Autodesk Inventor part; units mm, degrees
ref_plane "mss_or_XY" through (0, 0, 0) normal (1, 0, 0) x (0, 0, -1)
ref_plane "mss_or_YZ" through (0, 0, 0) normal (0, 0, -1) x (0, 1, 0)
ref_plane "mss_or_ZX" through (0, 0, 0) normal (0, 1, 0) x (1, 0, 0)
sketch "Sketch_3" plane through (0, 0, 0) normal (0, 0, 1) x (1, 0, 0)
  line L0 (6, 0) -> (0, 0)
  line L1 (0, 7.964) -> (0.135, 7.964)
  line L2 (0.135, 7.964) -> (0.135, 7.58)
  line L3 (0.135, 7.58) -> (1.5901, 7.58)
  arc A0 (4.4099, 7.58) -> (1.5901, 7.58) centre (3, 6.5) ccw
  line L4 (4.4099, 7.58) -> (5.865, 7.58)
  line L5 (5.865, 7.58) -> (5.865, 7.964)
  line L6 (5.865, 7.964) -> (6, 7.964)
  line L7 (6, 7.964) -> (6, 9.2)
  arc A1 (6, 9.2) -> (5.7, 9.5) centre (5.7, 9.2) ccw
  line L8 (5.7, 9.5) -> (0.3, 9.5)
  arc A2 (0.3, 9.5) -> (0, 9.2) centre (0.3, 9.2) ccw
  line L9 (0, 9.2) -> (0, 7.964)
revolve "Revolution1" add sketch "Sketch_3" angle 360 about axis through (6, 0, 0) along (1, 0, 0)
ref_plane "mss_or_XY" through (0, 0, 0) normal (1, 0, 0) x (0, 0, -1)
ref_plane "mss_or_YZ" through (0, 0, 0) normal (0, 0, -1) x (0, 1, 0)
ref_plane "mss_or_ZX" through (0, 0, 0) normal (0, 1, 0) x (1, 0, 0)
ref_plane "mss_or11_XY" through (6, 0, 0) normal (1, 0, 0) x (0, 0, -1)
ref_plane "mss_or11_YZ" through (6, 0, 0) normal (0, 0, -1) x (0, 1, 0)
ref_plane "mss_or11_ZX" through (6, 0, 0) normal (0, 1, 0) x (1, 0, 0)
ref_plane "mss_or2_1_XY" through (3, 6.5, 0) normal (1, 0, 0) x (0, 0, -1)
ref_plane "mss_or2_1_YZ" through (3, 6.5, 0) normal (0, 0, -1) x (0, 1, 0)
ref_plane "mss_or2_1_ZX" through (3, 6.5, 0) normal (0, 1, 0) x (1, 0, 0)
ref_plane "mss_or2_2_XY" through (3, 4.0527, 5.0819) normal (1, 0, 0) x (0, 0, -1)
ref_plane "mss_or2_2_YZ" through (3, 4.0527, 5.0819) normal (0, 0, -1) x (0, 1, 0)
ref_plane "mss_or2_2_ZX" through (3, 4.0527, 5.0819) normal (0, 1, 0) x (1, 0, 0)
ref_plane "mss_or2_3_XY" through (3, -1.4464, 6.337) normal (1, 0, 0) x (0, 0, -1)
ref_plane "mss_or2_3_YZ" through (3, -1.4464, 6.337) normal (0, 0, -1) x (0, 1, 0)
ref_plane "mss_or2_3_ZX" through (3, -1.4464, 6.337) normal (0, 1, 0) x (1, 0, 0)
ref_plane "mss_or2_4_XY" through (3, -5.8563, 2.8202) normal (1, 0, 0) x (0, 0, -1)
ref_plane "mss_or2_4_YZ" through (3, -5.8563, 2.8202) normal (0, 0, -1) x (0, 1, 0)
ref_plane "mss_or2_4_ZX" through (3, -5.8563, 2.8202) normal (0, 1, 0) x (1, 0, 0)
ref_plane "mss_or2_5_XY" through (3, -5.8563, -2.8202) normal (1, 0, 0) x (0, 0, -1)
ref_plane "mss_or2_5_YZ" through (3, -5.8563, -2.8202) normal (0, 0, -1) x (0, 1, 0)
ref_plane "mss_or2_5_ZX" through (3, -5.8563, -2.8202) normal (0, 1, 0) x (1, 0, 0)
ref_plane "mss_or2_6_XY" through (3, -1.4464, -6.337) normal (1, 0, 0) x (0, 0, -1)
ref_plane "mss_or2_6_YZ" through (3, -1.4464, -6.337) normal (0, 0, -1) x (0, 1, 0)
ref_plane "mss_or2_6_ZX" through (3, -1.4464, -6.337) normal (0, 1, 0) x (1, 0, 0)
ref_plane "mss_or2_7_XY" through (3, 4.0527, -5.0819) normal (1, 0, 0) x (0, 0, -1)
ref_plane "mss_or2_7_YZ" through (3, 4.0527, -5.0819) normal (0, 0, -1) x (0, 1, 0)
ref_plane "mss_or2_7_ZX" through (3, 4.0527, -5.0819) normal (0, 1, 0) x (1, 0, 0)
ref_plane "mss_or21_1_XY" through (3, 6.5, 0) normal (1, 0, 0) x (0, 0, -1)
ref_plane "mss_or21_1_YZ" through (3, 6.5, 0) normal (0, 0, -1) x (0, 1, 0)
ref_plane "mss_or21_1_ZX" through (3, 6.5, 0) normal (0, 1, 0) x (1, 0, 0)
ref_plane "mss_or21_2_XY" through (3, 4.0527, 5.0819) normal (1, 0, 0) x (0, 0, -1)
ref_plane "mss_or21_2_YZ" through (3, 4.0527, 5.0819) normal (0, 0, -1) x (0, 1, 0)
ref_plane "mss_or21_2_ZX" through (3, 4.0527, 5.0819) normal (0, 1, 0) x (1, 0, 0)
ref_plane "mss_or21_3_XY" through (3, -1.4464, 6.337) normal (1, 0, 0) x (0, 0, -1)
ref_plane "mss_or21_3_YZ" through (3, -1.4464, 6.337) normal (0, 0, -1) x (0, 1, 0)
ref_plane "mss_or21_3_ZX" through (3, -1.4464, 6.337) normal (0, 1, 0) x (1, 0, 0)
ref_plane "mss_or21_4_XY" through (3, -5.8563, 2.8202) normal (1, 0, 0) x (0, 0, -1)
ref_plane "mss_or21_4_YZ" through (3, -5.8563, 2.8202) normal (0, 0, -1) x (0, 1, 0)
ref_plane "mss_or21_4_ZX" through (3, -5.8563, 2.8202) normal (0, 1, 0) x (1, 0, 0)
ref_plane "mss_or21_5_XY" through (3, -5.8563, -2.8202) normal (1, 0, 0) x (0, 0, -1)
ref_plane "mss_or21_5_YZ" through (3, -5.8563, -2.8202) normal (0, 0, -1) x (0, 1, 0)
ref_plane "mss_or21_5_ZX" through (3, -5.8563, -2.8202) normal (0, 1, 0) x (1, 0, 0)
ref_plane "mss_or21_6_XY" through (3, -1.4464, -6.337) normal (1, 0, 0) x (0, 0, -1)
ref_plane "mss_or21_6_YZ" through (3, -1.4464, -6.337) normal (0, 0, -1) x (0, 1, 0)
ref_plane "mss_or21_6_ZX" through (3, -1.4464, -6.337) normal (0, 1, 0) x (1, 0, 0)
ref_plane "mss_or21_7_XY" through (3, 4.0527, -5.0819) normal (1, 0, 0) x (0, 0, -1)
ref_plane "mss_or21_7_YZ" through (3, 4.0527, -5.0819) normal (0, 0, -1) x (0, 1, 0)
ref_plane "mss_or21_7_ZX" through (3, 4.0527, -5.0819) normal (0, 1, 0) x (1, 0, 0)
properties part number "607ZZ Outer ring"
Source: CAD feature listing. Evaluate the final solid. Frame: model axes, mm. Round coordinates to 2 decimals unless told otherwise and drop trailing zeros. Loops run counter-clockwise (first coordinate to the right, second up) from the corner with the lowest first, then second, coordinate; pieces in that order, holes last. Notation, with made-up numbers: M -17.75,-30.75 L 28.25,-30.75 A27 cw 28.25,-3.75 Z; hole C 69.25,-14.5 d4. An arc over 180 degrees is marked long. Put each result on its own line as item: value.
(1) Ray query, line 1 (Z direction, x = 0.9, y = 0); line 2 (Z direction, x = 3.95, y = -1.5); line 3 (Y direction, x = 3.6, z = -5.75). Return the intervals inside material, ascending. Write a range as [from, to].
Solutions:
line 1: [-9.5, -7.58], [7.58, 9.5]
line 2: [-9.38, -7.86], [7.86, 9.38]
line 3: [-7.56, -5.81], [5.81, 7.56]
(2) Section C-C, the plane x = 4.95. Return loops of the section in (y, z), and give its area (3 significant figures).
Solutions:
outline: C 0,0 d19; hole C 0,0 d15.16
area: 103 mm²
(3) Pull-direction query (Z, two-part tool) for faces 1 (the face through (6, -3, 8)), 2 (the face through (0.87, 7.23, 2.28)), 3 (the face through (2.96, 4.38, 8.43)); classes: released by +Z, released by -Z, zero draft, split by the parting line, or undercut.
Solutions:
face 1: zero draft
face 2: undercut
face 3: split by the parting line
(4) Section A-A, the plane y = 0. Return loops of the section in (x, z) (3 decimals), and give its area (3 significant figures).
Solutions:
outline: M 0,-9.2 A0.3 ccw 0.3,-9.5 L 5.7,-9.5 A0.3 ccw 6,-9.2 L 6,-7.964 L 5.865,-7.964 L 5.865,-7.58 L 4.41,-7.58 A1.776 cw 1.59,-7.58 L 0.135,-7.58 L 0.135,-7.964 L 0,-7.964 Z; M 0,7.964 L 0.135,7.964 L 0.135,7.58 L 1.59,7.58 A1.776 cw 4.41,7.58 L 5.865,7.58 L 5.865,7.964 L 6,7.964 L 6,9.2 A0.3 ccw 5.7,9.5 L 0.3,9.5 A0.3 ccw 0,9.2 Z
area: 20.0 mm²
(5) Section D-D, the plane x = 3.8. Return loops of the section in (y, z), and give its area (3 significant figures).
Solutions:
outline: C 0,0 d19; hole C 0,0 d16.17
area: 78.1 mm²
